Can you work these out from the drawing? Everything is in mm from the part's minimum corner. A direction names the side the tool comes from. Give positions to 0.01 mm unless a question says otherwise; leave off trailing zeros. Order: outer loops, then holes, each group sorted by start corner. A loop starts at its lowest first (then second) coordinate and runs counter-clockwise, first axis right, second up. Notation, with made-up numbers: (80, -20) -> (115, -20) arc R11 ccw to (115, -6) -> close; hole circle Ø11 at (12, 73). An arc over 180 degrees is marked (long way). One line per item, written item: value.
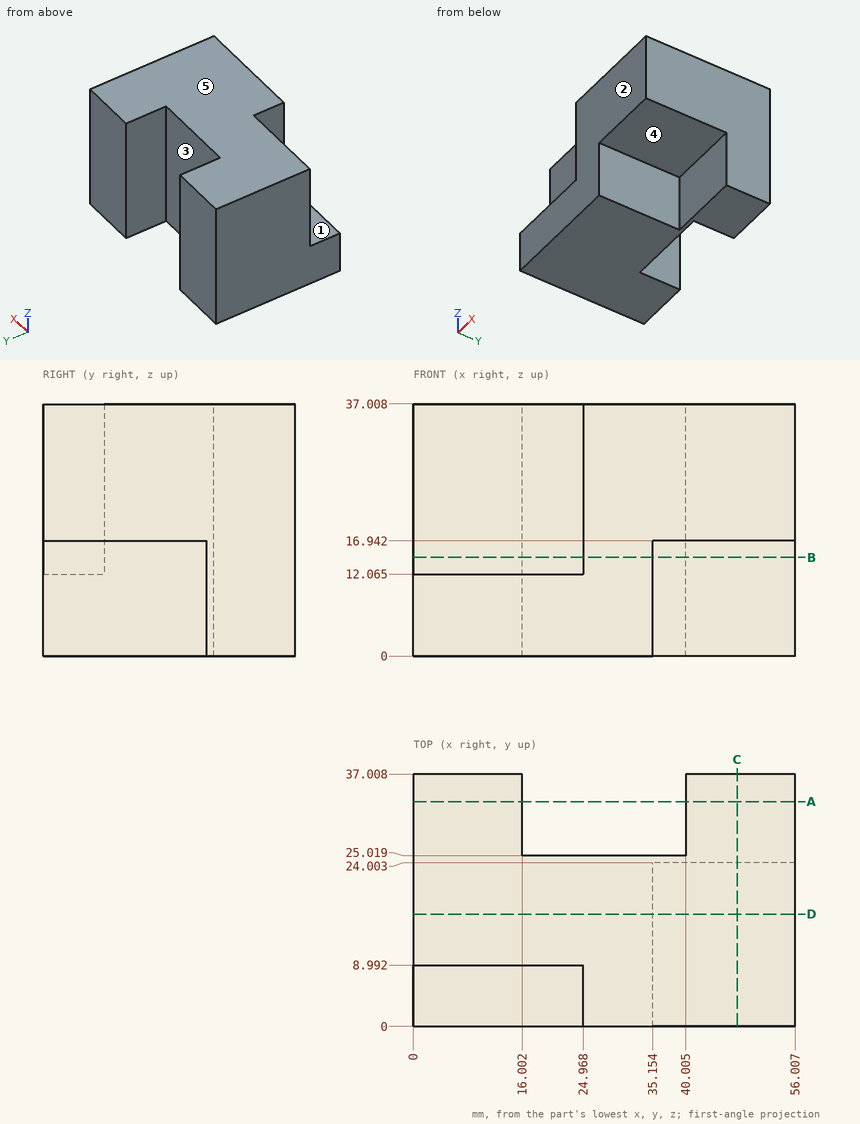
1) Suppose I cut it at D-D, the plane y = 16.5. Write out the boundary of the cut face in (x, z), then the cut area to 3 significant figures.
Answer below:
outline: (0, 0) -> (35.15, 0) -> (35.15, 16.94) -> (56.01, 16.94) -> (56.01, 37.01) -> (0, 37.01) -> close
area: 1,720 mm2
2) Suppose I cut it at A-A, the plane y = 33. Write out the boundary of the cut face in (x, z) (1 decimal), then the cut area to 3 significant figures.
Answer below:
outline: (0, 0) -> (16, 0) -> (16, 37) -> (0, 37) -> close; (40, 0) -> (56, 0) -> (56, 37) -> (40, 37) -> close
area: 1,180 mm2
3) Suppose I cut it at B-B, the plane z = 14.5. Write out the boundary of the cut face in (x, y) (1 decimal), then the cut area to 3 significant figures.
Answer below:
outline: (0, 9) -> (25, 9) -> (25, 0) -> (35.2, 0) -> (35.2, 24) -> (56, 24) -> (56, 37) -> (40, 37) -> (40, 25) -> (16, 25) -> (16, 37) -> (0, 37) -> close
area: 1,060 mm2
4) For the marked faces 1, 2, 3, 4 and 5, which set-ups out of +Z, -Z, +X, -X, +Y, -Y let a thin tool reach every point of the face, with its end or its side?
Answer below:
face 1: +Z, -X, -Y
face 2: +Z, -Z, +X, -X, -Y
face 3: +Z, -Z, +Y
face 4: -Z, +X, -Y
face 5: +Z, +X, -X, +Y, -Y
5) Suppose I cut it at C-C, the plane x = 47.5. Write out the boundary of the cut face in (y, z), then the cut area to 3 significant figures.
Answer below:
outline: (0, 16.94) -> (24, 16.94) -> (24, 0) -> (37.01, 0) -> (37.01, 37.01) -> (0, 37.01) -> close
area: 963 mm2
6) If I drill on line 1 along X through (y, z) = (33.5, 12) (1 decimal); line 2 along Z through (x, y) = (36.5, 21); line 3 along Y through (x, z) = (54.5, 15), over which ranges is the centre line in solid material (lowest first)?
Answer below:
line 1: x = 0 to 16, 40 to 56
line 2: z = 16.94 to 37.01
line 3: y = 24 to 37.01
7) For P1, Ø5, axis at y = 8, z = 9.5, coming from the +X side; P2, Ø12.5, axis at x = 15.5, z = 22.5, coming from the -Y side; P3, Ø12, axis at x = 31, z = 15.5, coming from the +Y side, each with a flat end and sliding along its axis, tell me the tip position at first contact or that it passes through.
Answer below:
P1: stops at x = 35.15
P2: stops at y = 8.99
P3: stops at y = 25.02
